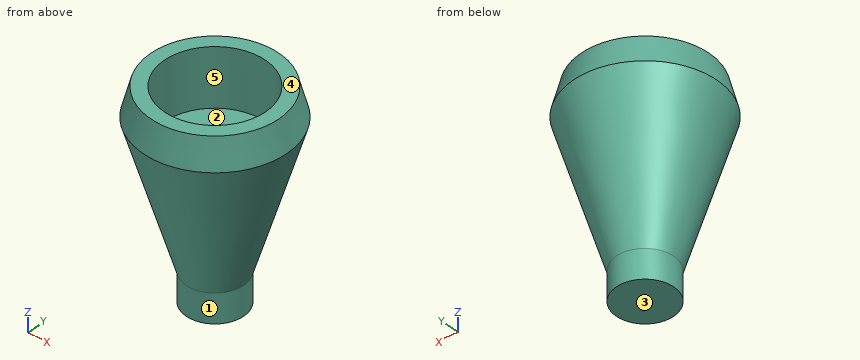
```python
from build123d import *

# Parameters (mm, degrees)
F2_R     = 4.826
F3_DEPTH = 38.1
F2_R_2   = 11.176
F4_DEPTH = 12.7


with BuildPart() as f1:
    # F0 (on Front) → F1 (revolve)
    with BuildSketch(Plane.XZ):
        Polygon((14.516552, 44.45), (14.516552, 0), (20.866552, 0), (20.866552, 6.35), (30.391552, 38.1), (28.690075, 44.45), align=None)
    revolve(axis=Axis((14.516552, 0, 22.225), (0, 0, -1)))

    # F2 (on face) → F3 (cut)
    with BuildSketch(Plane.XY.offset(44.45)):
        with Locations((14.516552, 0)):
            Circle(F2_R)
    extrude(amount=-F3_DEPTH, mode=Mode.SUBTRACT)

    # F2 (on face) → F4 (cut)
    with BuildSketch(Plane.XY.offset(44.45)):
        with Locations((14.516552, 0)):
            Circle(F2_R_2)
        with Locations((14.516552, 0)):
            Circle(F2_R, mode=Mode.SUBTRACT)
    extrude(amount=-F4_DEPTH, mode=Mode.SUBTRACT)


solid = f1.part
```
The listing builds one solid part. Answer for the finished solid, in the listing's coordinates (mm). Face numbers are marked on the shaded views. A direction names the side the tool comes from. Give positions to 0.01 mm unless a question says otherwise; leave off trailing zeros. Write each loop counter-clockwise with the first axis right and the second up, starting at its lowest first coordinate (ties: lowest second). Pieces come first, ordered by that corner, then holes. Notation, with made-up numbers: M 12,7 L 37,7 A10 ccw 37,24 Z; hole C 76,82.5 d1. An arc over 180 degrees is marked long. Write each question's results on one line, items separated by ' | '.
Q1. For a pull along Y with two mould halves and no side action, classify the marked faces 1, 2 and 3 as released by +Y, released by -Y, zero draft, split by the parting line, or undercut.
Output values:
face 1: split by the parting line | face 2: undercut | face 3: zero draft
Q2. Section C-C, the plane z = 32.5 is taken. Write down the section's boundary in (x, y) (3 decimals), then the cut area to 3 significant figures.
Output values:
outline: C 14.517,0 d28.39; hole C 14.517,0 d22.352 | area: 241 mm2
Q3. Section A-A, the plane y = 0 is taken. Write down the section's boundary in (x, z), then the cut area to 3 significant figures.
Output values:
outline: M -1.36,38.1 L 8.17,6.35 L 8.17,0 L 20.87,0 L 20.87,6.35 L 30.39,38.1 L 28.69,44.45 L 25.69,44.45 L 25.69,31.75 L 19.34,31.75 L 19.34,6.35 L 9.69,6.35 L 9.69,31.75 L 3.34,31.75 L 3.34,44.45 L 0.34,44.45 Z | area: 448 mm2
Q4. Section B-B, the plane z = 26 is taken. Write down the section's boundary in (x, y) (3 decimals).
Output values:
outline: C 14.517,0 d24.49; hole C 14.517,0 d9.652
Q5. Consider L1, parallel to Y at x = 14, z = 14; L2, parallel to Y at x = 20, z = 32; L3, parallel to Z at x = 15, y = -4. Determine where each line is inside the solid, lowest interval first. Write a range as from..to.
Output values:
L1: -8.63..-4.8, 4.8..8.63 | L2: -12.93..-9.74, 9.74..12.93 | L3: 0..6.35
Q6. Flat-ended cylindrical pins translate along their axes: P1, Ø12, axis at y = -4, z = 29, coming from the +X side; P2, Ø1.5, axis at x = 14, z = 21.5, coming from the +Y side; P3, Ø4, axis at x = 17.5, z = 36.5, coming from the -Y side. Find the tip coordinate at first contact, or state that the pin passes through.
Output values:
P1: x = 29.23 | P2: y = 11.11 | P3: y = -15.77
Q7. A tool of negligible diameter and unlimited length cuts with its end or side. For the marked faces 4 and 5, from which of +Z, -Z, +X, -X, +Y, -Y can it reach the whole face along a straight path? Write none if from no direction.
Output values:
face 4: +Z, +X, -X, +Y, -Y | face 5: +Z
